```python
from build123d import *

# Parameters (mm, degrees)
BOSS_EXTRUDE1_DEPTH = 7.8
SKETCH2_R           = 3.995
BOSS_EXTRUDE2_DEPTH = 78
CUT_EXTRUDE1_START  = -1
SKETCH3_R           = 5
SKETCH3_R_2         = 3.8
CUT_EXTRUDE1_DEPTH  = 0.9


with BuildPart() as part:
    # Sketch1 → Boss-Extrude1 (new body)
    with BuildSketch(Plane(origin=(0, 0, 0), x_dir=(0, 0, -1), z_dir=(1, 0, 0))):
        with BuildLine():
            Line((1.985, 3.466958321), (1.985, -3.466958321))
            ThreePointArc((1.985, -3.466958321), (-3.995, 0), (1.985, 3.466958321))
        make_face()
    extrude(amount=BOSS_EXTRUDE1_DEPTH)

    # Sketch2 → Boss-Extrude2 (add)
    with BuildSketch(Plane(origin=(7.8, 0, 0), x_dir=(0, 0, -1), z_dir=(1, 0, 0))):
        with Locations(Location((0, 0, 0), (0, 0, 299.79320791))):
            Circle(SKETCH2_R)
    extrude(amount=BOSS_EXTRUDE2_DEPTH)

    # Sketch3 → Cut-Extrude1 (cut)
    with BuildSketch(Plane(origin=(85.8, 0, 0), x_dir=(0, 0, -1), z_dir=(1, 0, 0)).offset(CUT_EXTRUDE1_START)):
        Circle(SKETCH3_R)
        Circle(SKETCH3_R_2, mode=Mode.SUBTRACT)
    extrude(amount=-CUT_EXTRUDE1_DEPTH, mode=Mode.SUBTRACT)

    # Cut-Extrude2 cone 1 section (through the dimple's axis) → Cut-Extrude2 (revolve, cut)
    with BuildSketch(Plane(origin=(43.434, 0, -3.995), x_dir=(0, 1, 0), z_dir=(1, 0, 0))):
        Polygon((0, 0), (1.778, 0), (0, 1.778), align=None)
    revolve(axis=Axis((43.434, 0, -3.995), (0, 0, 1)), mode=Mode.SUBTRACT)


solid = part.part
```
Geometry check sheet. Reference: the model listing, model coordinates, mm. A direction names the side the tool comes from. Round coordinates to 2 decimals unless told otherwise and drop trailing zeros. Loops run counter-clockwise (first coordinate to the right, second up) from the corner with the lowest first, then second, coordinate; pieces in that order, holes last. Notation, with made-up numbers: M 65.5,79.5 L 101.5,79.5 A30 ccw 101.5,102.5 Z; hole C -26,88.25 d1. An arc over 180 degrees is marked long. Return JSON: item names as keys, results as strings. Group by question number.
(1) Section check A-A, the plane z = -3. Enter the section's corners in (x, y).
(2) Scan lines: line 1 along Z through (x, y) = (66, -2); line 2 along X through (y, z) = (0, -2.5); line 3 along X through (y, z) = (-1.25, -3.25). Record each from-to range of solid material in increasing order. Write a range as [from, to].
(3) Go/stop test with flat-tipped pins: pin 1 (2 mm diameter, centred on y = 1.5, z = -3.5, fed in from -X); pin 2 (1 mm diameter, centred on x = 17, y = 2.5, fed in from +Z); pin 3 (1 mm diameter, centred on x = 48, z = -3, fed in from -Y). Record where each tip stops, or that it passes through.
(4) Section check B-B, the plane x = 46. Enter the section's corners in (y, z) (3 decimals).
(5) Set-up check for faces 1 (the face through (84.356, 0.167, 3.796)), 2 (the face through (85.8, 0, 0)), 3 (the face through (7.8, 0, -3)): record each of +Z, -Z, +X, -X, +Y, -Y from which the full face is reachable in a straight line by a thin tool's end or side.
(6) Mould release check, pull along Y, two halves, no side actions. Record for faces 4 (the face through (43.618, 0.445, -2.698)), 5 (the face through (4, 0, -1.985)), 6 (the face through (85.29, 2.42, -3.18)): pulls with the +Y half, pulls with the -Y half, needs draft (parallel to the pull), parting line crosses it, or undercut.
Data:
{
 "1": {"outline": "M 7.8,-2.64 L 83.9,-2.64 L 83.9,-2.33 L 84.8,-2.33 L 84.8,-2.64 L 85.8,-2.64 L 85.8,2.64 L 84.8,2.64 L 84.8,2.33 L 83.9,2.33 L 83.9,2.64 L 7.8,2.64 Z; hole C 43.43,0 d1.57"},
 "2": {"line 1": "[-3.46, 3.46]", "line 2": "[7.8, 43.15], [43.72, 85.8]", "line 3": "[7.8, 85.8]"},
 "3": {"pin 1": "x = 7.8", "pin 2": "z = 3.46", "pin 3": "y = -3.12"},
 "4": {"outline": "C 0,0 d7.99"},
 "5": {"face 1": "none", "face 2": "+Z, -Z, +X, +Y, -Y", "face 3": "-Z, -X, +Y, -Y"},
 "6": {"face 4": "undercut", "face 5": "needs draft", "face 6": "parting line crosses it"}
}
